```python
from build123d import *

# Parameters (mm, degrees)
SKETCH1_R             = 3.05
BOSS_EXTRUDE1_DEPTH   = 10
BOSS_EXTRUDE2_DEPTH   = 75.9
SKETCH3_R             = 1.4
CUT_EXTRUDE1_DEPTH    = 6
CHAMFER1_SIZE         = 1.55
CHAMFER2_SIZE         = 2
MIRROR1_START         = -85.9
MIRROR1_OUTLINE_R     = 1.4
MIRROR1_DEPTH         = 85.9
MIRROR1_START_2       = -10
MIRROR1_2_OUTLINE_W   = 195
MIRROR1_2_OUTLINE_H   = 100.5
MIRROR1_2_OUTLINE_R   = 3.05
MIRROR1_2_OUTLINE_R_2 = 1.4
MIRROR1_2_DEPTH       = 10
MIRROR1_START_3       = -79.9
MIRROR1_3_OUTLINE_R   = 1.4
MIRROR1_3_DEPTH       = 69.9
SKETCH4_W             = 135.019613606
SKETCH4_H             = 106.174514336
CUT_EXTRUDE2_DEPTH    = 236.5929965
SKETCH5_W             = 195
SKETCH5_H             = 0.5
CUT_EXTRUDE3_DEPTH    = 233.133711468
CHAMFER3_SIZE         = 3.1
CHAMFER4_SIZE         = 3.1


# Read off the part's stored shape, not the designer's step: Mirror1
with BuildPart() as part:
    # Sketch1 → Boss-Extrude1 (new body)
    with BuildSketch(Plane(origin=(0, 0, 0), x_dir=(1, 0, 0), z_dir=(0, 1, 0))):
        Polygon((0, 0), (195, 0), (195, 95), (195, 100.5), (0, 100.5), (0, 95), align=None)
        with Locations(Location((10, 85, 0), (0, 0, 270))):
            Circle(SKETCH1_R, mode=Mode.SUBTRACT)
        with Locations(Location((185, 85, 0), (0, 0, 90))):
            Circle(SKETCH1_R, mode=Mode.SUBTRACT)
        with Locations(Location((185, 10, 0), (0, 0, 270))):
            Circle(SKETCH1_R, mode=Mode.SUBTRACT)
        with Locations(Location((10, 10, 0), (0, 0, 90))):
            Circle(SKETCH1_R, mode=Mode.SUBTRACT)
    extrude(amount=BOSS_EXTRUDE1_DEPTH)

    # Sketch2 → Boss-Extrude2 (add)
    with BuildSketch(Plane(origin=(0, 10, 0), x_dir=(1, 0, 0), z_dir=(0, 1, 0))):
        with BuildLine():
            Line((43.7, 59), (91.1, 59))
            Line((91.1, 59), (91.1, 45.6))
            Line((91.1, 45.6), (158, 45.6))
            Line((158, 45.6), (158, 39.6))
            Line((158, 39.6), (166, 39.6))
            Line((166, 39.6), (166, 9.6))
            Line((166, 9.6), (158, 9.6))
            Line((158, 9.6), (158, 3.6))
            Line((158, 3.6), (41.7, 3.6))
            Line((41.7, 3.6), (41.7, 9.6))
            Line((41.7, 9.6), (33.7, 9.6))
            Line((33.7, 9.6), (33.7, 39.6))
            Line((33.7, 39.6), (41.7, 39.6))
            Line((41.7, 39.6), (41.7, 57))
            ThreePointArc((41.7, 57), (42.285786438, 58.414213562), (43.7, 59))
        make_face()
    extrude(amount=BOSS_EXTRUDE2_DEPTH)

    # Sketch3 → Cut-Extrude1 (cut)
    with BuildSketch(Plane(origin=(0, 85.9, 0), x_dir=(1, 0, 0), z_dir=(0, 1, 0))):
        with Locations(Location((37.7, 32.1, 0), (0, 0, 270))):
            Circle(SKETCH3_R)
        with Locations(Location((37.7, 17.1, 0), (0, 0, 90))):
            Circle(SKETCH3_R)
        with Locations(Location((162, 17.1, 0), (0, 0, 270))):
            Circle(SKETCH3_R)
        with Locations(Location((162, 32.1, 0), (0, 0, 90))):
            Circle(SKETCH3_R)
    extrude(amount=-CUT_EXTRUDE1_DEPTH, mode=Mode.SUBTRACT)

    # Chamfer1
    chamfer1_edges = [part.edges().sort_by_distance(p)[0] for p in [
        (41.7, 47.95, -39.6),
        (33.7, 47.95, -39.6),
        (33.7, 47.95, -9.6),
        (41.7, 47.95, -9.6),
        (158, 47.95, -9.6),
        (166, 47.95, -9.6),
        (166, 47.95, -39.6),
        (158, 47.95, -39.6),
    ]]
    chamfer(chamfer1_edges, length=CHAMFER1_SIZE)

    # Chamfer2
    chamfer2_edges = [part.edges().sort_by_distance(p)[0] for p in [
        (41.7, 47.95, -3.6),
        (158, 47.95, -3.6),
        (158, 47.95, -45.6),
    ]]
    chamfer(chamfer2_edges, length=CHAMFER2_SIZE)

    # Mirror1 outline → Mirror1 (add)
    with BuildSketch(Plane(origin=(0, 0, 0), x_dir=(1, 0, 0), z_dir=(0, 1, 0)).offset(MIRROR1_START)):
        with BuildLine():
            Line((91.1, 59), (43.7, 59))
            ThreePointArc((43.7, 59), (42.285786438, 58.414213562), (41.7, 57))
            Line((41.7, 57), (41.7, 41.15))
            Line((41.7, 41.15), (40.15, 39.6))
            Line((40.15, 39.6), (35.25, 39.6))
            Line((35.25, 39.6), (33.7, 38.05))
            Line((33.7, 38.05), (33.7, 11.15))
            Line((33.7, 11.15), (35.25, 9.6))
            Line((35.25, 9.6), (40.15, 9.6))
            Line((40.15, 9.6), (41.7, 8.05))
            Line((41.7, 8.05), (41.7, 5.6))
            Line((41.7, 5.6), (43.7, 3.6))
            Line((43.7, 3.6), (156, 3.6))
            Line((156, 3.6), (158, 5.6))
            Line((158, 5.6), (158, 8.05))
            Line((158, 8.05), (159.55, 9.6))
            Line((159.55, 9.6), (164.45, 9.6))
            Line((164.45, 9.6), (166, 11.15))
            Line((166, 11.15), (166, 38.05))
            Line((166, 38.05), (164.45, 39.6))
            Line((164.45, 39.6), (159.55, 39.6))
            Line((159.55, 39.6), (158, 41.15))
            Line((158, 41.15), (158, 43.6))
            Line((158, 43.6), (156, 45.6))
            Line((156, 45.6), (91.1, 45.6))
            Line((91.1, 45.6), (91.1, 59))
        make_face()
        with Locations((37.7, 17.1)):
            Circle(MIRROR1_OUTLINE_R, mode=Mode.SUBTRACT)
        with Locations((37.7, 32.1)):
            Circle(MIRROR1_OUTLINE_R, mode=Mode.SUBTRACT)
        with Locations((162, 17.1)):
            Circle(MIRROR1_OUTLINE_R, mode=Mode.SUBTRACT)
        with Locations((162, 32.1)):
            Circle(MIRROR1_OUTLINE_R, mode=Mode.SUBTRACT)
    extrude(amount=MIRROR1_DEPTH)

    # Mirror1 2 outline → Mirror1 2 (add)
    # profile 1 of 5: a face of its own
    with BuildSketch(Plane(origin=(0, 0, 0), x_dir=(1, 0, 0), z_dir=(0, 1, 0)).offset(MIRROR1_START_2)):
        with Locations((97.5, 50.25)):
            Rectangle(MIRROR1_2_OUTLINE_W, MIRROR1_2_OUTLINE_H)
        with Locations((10, 10)):
            Circle(MIRROR1_2_OUTLINE_R, mode=Mode.SUBTRACT)
        with Locations((185, 10)):
            Circle(MIRROR1_2_OUTLINE_R, mode=Mode.SUBTRACT)
        with BuildLine():
            ThreePointArc((41.7, 57), (42.285786438, 58.414213562), (43.7, 59))
            Line((43.7, 59), (91.1, 59))
            Line((91.1, 59), (91.1, 45.6))
            Line((91.1, 45.6), (156, 45.6))
            Line((156, 45.6), (158, 43.6))
            Line((158, 43.6), (158, 41.15))
            Line((158, 41.15), (159.55, 39.6))
            Line((159.55, 39.6), (164.45, 39.6))
            Line((164.45, 39.6), (166, 38.05))
            Line((166, 38.05), (166, 11.15))
            Line((166, 11.15), (164.45, 9.6))
            Line((164.45, 9.6), (159.55, 9.6))
            Line((159.55, 9.6), (158, 8.05))
            Line((158, 8.05), (158, 5.6))
            Line((158, 5.6), (156, 3.6))
            Line((156, 3.6), (43.7, 3.6))
            Line((43.7, 3.6), (41.7, 5.6))
            Line((41.7, 5.6), (41.7, 8.05))
            Line((41.7, 8.05), (40.15, 9.6))
            Line((40.15, 9.6), (35.25, 9.6))
            Line((35.25, 9.6), (33.7, 11.15))
            Line((33.7, 11.15), (33.7, 38.05))
            Line((33.7, 38.05), (35.25, 39.6))
            Line((35.25, 39.6), (40.15, 39.6))
            Line((40.15, 39.6), (41.7, 41.15))
            Line((41.7, 41.15), (41.7, 57))
        make_face(mode=Mode.SUBTRACT)
        with Locations((10, 85)):
            Circle(MIRROR1_2_OUTLINE_R, mode=Mode.SUBTRACT)
        with Locations((185, 85)):
            Circle(MIRROR1_2_OUTLINE_R, mode=Mode.SUBTRACT)
    # profile 2 of 5: a face of its own
    with BuildSketch(Plane(origin=(0, 0, 0), x_dir=(1, 0, 0), z_dir=(0, 1, 0)).offset(MIRROR1_START_2)):
        with Locations((37.7, 32.1)):
            Circle(MIRROR1_2_OUTLINE_R_2)
    # profile 3 of 5: a face of its own
    with BuildSketch(Plane(origin=(0, 0, 0), x_dir=(1, 0, 0), z_dir=(0, 1, 0)).offset(MIRROR1_START_2)):
        with Locations((37.7, 17.1)):
            Circle(MIRROR1_2_OUTLINE_R_2)
    # profile 4 of 5: a face of its own
    with BuildSketch(Plane(origin=(0, 0, 0), x_dir=(1, 0, 0), z_dir=(0, 1, 0)).offset(MIRROR1_START_2)):
        with Locations((162, 17.1)):
            Circle(MIRROR1_2_OUTLINE_R_2)
    # profile 5 of 5: a face of its own
    with BuildSketch(Plane(origin=(0, 0, 0), x_dir=(1, 0, 0), z_dir=(0, 1, 0)).offset(MIRROR1_START_2)):
        with Locations((162, 32.1)):
            Circle(MIRROR1_2_OUTLINE_R_2)
    extrude(amount=MIRROR1_2_DEPTH)

    # Mirror1 3 outline → Mirror1 3 (add)
    with BuildSketch(Plane(origin=(0, 0, 0), x_dir=(1, 0, 0), z_dir=(0, 1, 0)).offset(MIRROR1_START_3)):
        with Locations((37.7, 32.1)):
            Circle(MIRROR1_3_OUTLINE_R)
        with Locations((37.7, 17.1)):
            Circle(MIRROR1_3_OUTLINE_R)
        with Locations((162, 17.1)):
            Circle(MIRROR1_3_OUTLINE_R)
        with Locations((162, 32.1)):
            Circle(MIRROR1_3_OUTLINE_R)
    extrude(amount=MIRROR1_3_DEPTH)

    # Sketch4 → Cut-Extrude2 (cut, through all)
    with BuildSketch(Plane.ZY):
        with Locations((-58.433006885, 53.087257168)):
            Rectangle(SKETCH4_W, SKETCH4_H)
    extrude(amount=-CUT_EXTRUDE2_DEPTH, mode=Mode.SUBTRACT)

    # Sketch5 → Cut-Extrude3 (cut, through all)
    with BuildSketch(Plane.XZ.offset(10)):
        with Locations((97.5, -100.25)):
            Rectangle(SKETCH5_W, SKETCH5_H)
    extrude(amount=-CUT_EXTRUDE3_DEPTH, mode=Mode.SUBTRACT)

    # Chamfer3
    chamfer3_edges = [part.edges().sort_by_distance(p)[0] for p in [
        (6.95, -10, -10),
        (181.95, -10, -10),
        (181.95, -10, -85),
        (6.95, -10, -85),
    ]]
    chamfer(chamfer3_edges, length=CHAMFER3_SIZE)

    # Chamfer4
    chamfer4_edges = [part.edges().sort_by_distance(p)[0] for p in [
        (195, -10, -50),
        (97.5, -10, 0),
        (0, -5, 0),
        (195, -5, 0),
        (0, -10, -50),
        (0, -5, -100),
        (195, -5, -100),
        (97.5, -10, -100),
    ]]
    chamfer(chamfer4_edges, length=CHAMFER4_SIZE)


solid = part.part
```
Work out the finished part from the listing and answer in its coordinate system (mm). A direction names the side the tool comes from. Round coordinates to 2 decimals unless told otherwise and drop trailing zeros. Loops run counter-clockwise (first coordinate to the right, second up) from the corner with the lowest first, then second, coordinate; pieces in that order, holes last.
(1) Find the intervals of material crossed by L1, parallel to X at y = -81.3, z = -17.1; L2, parallel to X at y = -3, z = -85; L3, parallel to Z at x = 185, y = -3.25, in increasing order.
Computed values:
L1: x = 33.7 to 36.3, 39.1 to 160.6, 163.4 to 166
L2: x = 0 to 6.95, 13.05 to 181.95, 188.05 to 195
L3: z = -100 to -88.05, -81.95 to -13.05, -6.95 to 0
(2) For faces 1 (the flat face through (124, -48, -45.6)), 2 (the flat face through (38, -48, -9.6)), 3 (the flat face through (68, -48, -59)), determine the directions among +Z, -Z, +X, -X, +Y, -Y from which every point of the face is accessible in a straight line to the end or side of a thin tool.
Computed values:
face 1: -Z, +X, -Y
face 2: +Z, -X, -Y
face 3: -Z, +X, -X, -Y
(3) The part is cut by section D-D, the plane y = -31. Give the vertices of the cut face in (x, z).
Computed values:
outline: (33.7, -38.05) - (35.25, -39.6) - (40.15, -39.6) - (41.7, -41.15) - (41.7, -57) arc R2 ccw to (43.7, -59) - (91.1, -59) - (91.1, -45.6) - (156, -45.6) - (158, -43.6) - (158, -41.15) - (159.55, -39.6) - (164.45, -39.6) - (166, -38.05) - (166, -11.15) - (164.45, -9.6) - (159.55, -9.6) - (158, -8.05) - (158, -5.6) - (156, -3.6) - (43.7, -3.6) - (41.7, -5.6) - (41.7, -8.05) - (40.15, -9.6) - (35.25, -9.6) - (33.7, -11.15) - close
(4) The mould has two halves that part along Z. Classify faces 4 (the cylindrical face through (7.75, -3.5, -12.06)), 5 (the flat face through (33.7, -48, -25)), 6 (the flat face through (162, -48, -39.6)): pulls with the +Z half, pulls with the -Z half, needs draft (parallel to the pull), parting line crosses it, or undercut.
Computed values:
face 4: undercut
face 5: needs draft
face 6: pulls with the -Z half
(5) The part is cut by section A-A, the plane z = -85. Give the vertices of the cut face in (x, y), and give its area (3 significant figures).
Computed values:
outline: (0, -6.9) - (3.1, -10) - (3.85, -10) - (6.95, -6.9) - (6.95, 0) - (0, 0) - close; (13.05, -6.9) - (16.15, -10) - (178.85, -10) - (181.95, -6.9) - (181.95, 0) - (13.05, 0) - close; (188.05, -6.9) - (191.15, -10) - (191.9, -10) - (195, -6.9) - (195, 0) - (188.05, 0) - close
area: 1,800 mm2
(6) The part is cut by section B-B, the plane x = 10. Give the vertices of the cut face in (y, z), and give its area (3 significant figures).
Computed values:
outline: (-10, -96.9) - (-6.9, -100) - (0, -100) - (0, -88.05) - (-6.9, -88.05) - (-10, -91.15) - close; (-10, -78.85) - (-6.9, -81.95) - (0, -81.95) - (0, -13.05) - (-6.9, -13.05) - (-10, -16.15) - close; (-10, -3.85) - (-6.9, -6.95) - (0, -6.95) - (0, 0) - (-6.9, 0) - (-10, -3.1) - close
area: 849 mm2
(7) Each of these flat-tipped pins is pushed along its axis until it touches: P1, Ø1.4, axis at x = 162, z = -17, coming from the -Y side; P2, Ø4, axis at x = 161.5, y = -55.5, coming from the +Z side; P3, Ø1.2, axis at y = -31, z = -7, coming from the -X side. Where does it stop, or does it pass through?
Computed values:
P1: stops at y = -79.9
P2: stops at z = -9.55
P3: stops at x = 41.7
(8) The part is cut by section C-C, the plane z = -24. Give the vertices of the cut face in (x, y).
Computed values:
outline: (0, -6.9) - (3.1, -10) - (33.7, -10) - (33.7, -85.9) - (166, -85.9) - (166, -10) - (191.9, -10) - (195, -6.9) - (195, 0) - (0, 0) - close
